The figure shows three views and two pictorial views of one solid part (mm, origin at its lowest corner). Answer the questions. A direction names the side the tool comes from. Give positions to 0.01 mm unless a question says otherwise; leave off trailing zeros. Loops run counter-clockwise (first coordinate to the right, second up) from the corner with the lowest first, then second, coordinate; pieces in that order, holes last. Notation, with made-up numbers: (7.5, 74) - (31.5, 74) arc R13 ccw to (31.5, 80) - close; hole circle Ø8 at (10, 49). An arc over 180 degrees is marked (long way). Use CSV: the item, a comma, the result in double quotes.
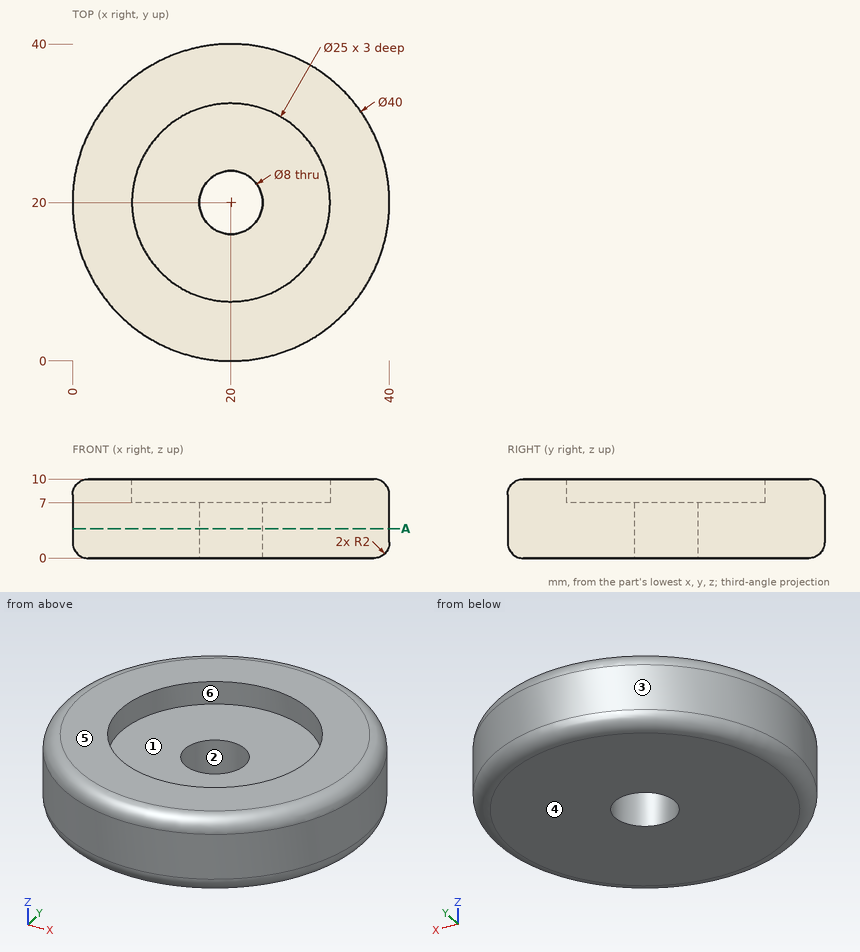
Item 1: Given P1, Ø4, axis at y = 31.5, z = 5.5, coming from the +X side; P2, Ø1.5, axis at x = 10, z = 4, coming from the -Y side; P3, Ø10.5, axis at x = 20, y = 20, coming from the +Z side, each flat-ended and moving along its own axis, determine where each tip first touches the part or whether it passes through.
Determined:
P1,"stops at x = 37.6"
P2,"stops at y = 2.27"
P3,"stops at z = 7"
Item 2: For the marked faces 5 and 6, determine the directions among +Z, -Z, +X, -X, +Y, -Y from which every point of the face is accessible in a straight line to the end or side of a thin tool.
Determined:
face 5,"+Z, +X, -X, +Y, -Y"
face 6,"+Z"
Item 3: Find the intervals of material crossed by line 1 (Y direction, x = 20, z = 7.75); line 2 (Z direction, x = 30, y = 19); line 3 (X direction, y = 24, z = 8), in increasing order.
Determined:
line 1,"y = 0 to 7.5, 32.5 to 40"
line 2,"z = 0 to 7"
line 3,"x = 0.4 to 8.16, 31.84 to 39.6"
Item 4: A cutting plane is placed at A-A on z = 3.75. Determine the outline of the cut face in (x, y), and give its area (3 significant figures).
Determined:
outline,"circle Ø40 at (20, 20); hole circle Ø8 at (20, 20)"
area,"1,210 mm²"
Item 5: The mould has two halves that part along Y. Classify the marked faces 1, 2, 3 and 4: pulls with the +Y half, pulls with the -Y half, needs draft (parallel to the pull), parting line crosses it, or undercut.
Determined:
face 1,"undercut"
face 2,"undercut"
face 3,"parting line crosses it"
face 4,"needs draft"
